from build123d import *

# Parameters (mm, degrees)
SKETCH1_R      = 3.15
EXTRUDE1_DEPTH = 4
CHAMFER1_SIZE  = 0.64


with BuildPart() as part:
    # Sketch1 → Extrude1 (new body)
    with BuildSketch(Plane.XY):
        Polygon((-23.945658648, 33.397892325), (-23.945658648, -41.602107675), (51.054341352, -41.602107675), (51.054341352, -16.602107675), (1.054341352, 33.397892325), align=None)
        with Locations((-11.445658648, -29.102107675)):
            Circle(SKETCH1_R, mode=Mode.SUBTRACT)
        with Locations((-11.445658648, -4.102107675)):
            Circle(SKETCH1_R, mode=Mode.SUBTRACT)
        with Locations((-11.445658648, 20.897892325)):
            Circle(SKETCH1_R, mode=Mode.SUBTRACT)
        with Locations((13.554341352, -29.102107675)):
            Circle(SKETCH1_R, mode=Mode.SUBTRACT)
        with Locations((38.554341352, -29.102107675)):
            Circle(SKETCH1_R, mode=Mode.SUBTRACT)
    extrude(amount=EXTRUDE1_DEPTH)

    # Chamfer1
    chamfer1_edges = [part.edges().sort_by_distance(p)[0] for p in [
        (51.054341352, -29.102107675, 4),
        (26.054341352, 8.397892325, 4),
        (26.054341352, 8.397892325, 0),
        (51.054341352, -29.102107675, 0),
        (-23.945658648, -4.102107675, 0),
        (-23.945658648, -4.102107675, 4),
    ]]
    chamfer(chamfer1_edges, length=CHAMFER1_SIZE)


solid = part.part
Model file for the job. Use its own axes, mm. Round coordinates to 2 decimals unless told otherwise and drop trailing zeros. Order: outer loops, then holes, each group sorted by start corner. A loop starts at its lowest first (then second) coordinate and runs counter-clockwise, first axis right, second up.
(1) Band-saw the part on C-C (z = 2.75). List the corners of the cut face in (x, y).
(2) Pull direction Y, two halves, no side cores. Call faces 1 (the face through (13, -41.602, 2)), 2 (the face through (-8.44, -3.16, 1.97)), 3 (the face through (26.4, 8.05, 1.98)), 4 (the face through (-23.946, -4, 2)): released by +Y, released by -Y, zero draft, split by the parting line, or undercut.
(3) Band-saw the part on B-B (x = 40). List the corners of the cut face in (y, z), then the cut area to 3 significant figures.
(4) Band-saw the part on A-A (y = 20). List the corners of the cut face in (x, z).
(5) Drill centre lines: line 1 (Y direction, x = -11, z = 3.1); line 2 (X direction, y = -31, z = 2.65); line 3 (Y direction, x = 12.5, z = 3.1). Where is each one in solid material? Low to high.
(6) Pin check, flat tips, straight feed: pin 1 (8 mm diameter, centred on x = -11.45, y = -29.1, fed in from -Z); pin 2 (5 mm diameter, centred on x = -11.45, y = -4.1, fed in from -Z). Stop position of each tip, or through.
(7) Band-saw the part on D-D (y = 0.5). List the corners of the cut face in (x, z), then the cut area to 3 significant figures.
Verdict:
1. outline: (-23.95, -41.6) - (51.05, -41.6) - (51.05, -16.6) - (1.05, 33.4) - (-23.95, 33.4) - close; hole circle Ø6.3 at (-11.45, -29.1); hole circle Ø6.3 at (-11.45, -4.1); hole circle Ø6.3 at (-11.45, 20.9); hole circle Ø6.3 at (13.55, -29.1); hole circle Ø6.3 at (38.55, -29.1)
2. face 1: released by -Y
2. face 2: undercut
2. face 3: released by +Y
2. face 4: zero draft
3. outline: (-41.6, 0) - (-31.9, 0) - (-31.9, 4) - (-41.6, 4) - close; (-26.3, 0) - (-6.45, 0) - (-5.55, 0.64) - (-5.55, 3.36) - (-6.45, 4) - (-26.3, 4) - close
3. area: 121 mm2
4. outline: (-23.95, 0.64) - (-23.31, 0) - (-14.46, 0) - (-14.46, 4) - (-23.31, 4) - (-23.95, 3.36) - close; (-8.43, 0) - (13.55, 0) - (14.45, 0.64) - (14.45, 3.36) - (13.55, 4) - (-8.43, 4) - close
5. line 1: y = -41.6 to -32.22, -25.98 to -7.22, -0.98 to 17.78, 24.02 to 33.4
5. line 2: x = -23.95 to -13.96, -8.93 to 11.04, 16.07 to 36.04, 41.07 to 51.05
5. line 3: y = -41.6 to -32.07, -26.13 to 21.95
6. pin 1: stops at z = 0
6. pin 2: passes through
7. outline: (-23.95, 0.64) - (-23.31, 0) - (33.05, 0) - (33.95, 0.64) - (33.95, 3.36) - (33.05, 4) - (-23.31, 4) - (-23.95, 3.36) - close
7. area: 231 mm2
